Geometry check sheet. Reference: drawing and pictorial views, mm from the part's lowest x, y, z. Give positions to 0.01 mm unless a question says otherwise; leave off trailing zeros. Loops run counter-clockwise (first coordinate to the right, second up) from the corner with the lowest first, then second, coordinate; pieces in that order, holes last. Notation, with made-up numbers: M 59.5,87.25 L 101.5,87.25 A18 ccw 101.5,100.25 Z; hole C -24,13 d9. An arc over 180 degrees is marked long. Put each result on its own line as item: value. Start each with the question number.
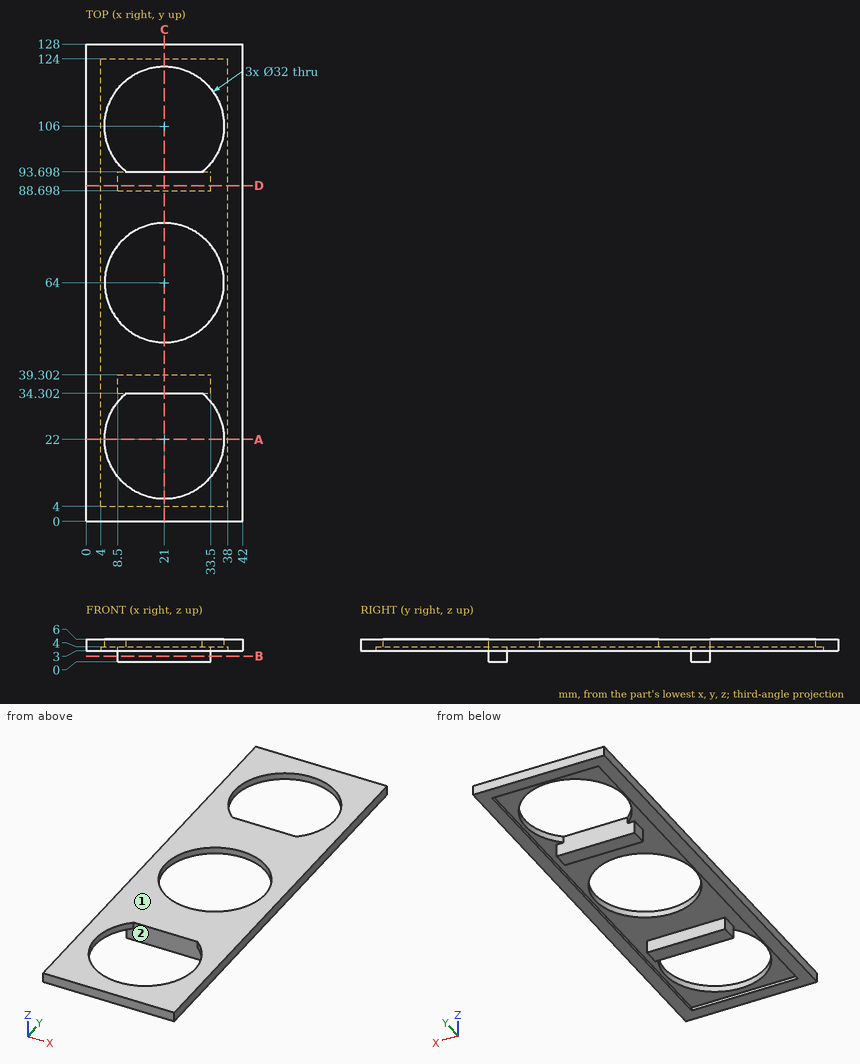
Q1. Section check D-D, the plane y = 90. Record the cut outline in (x, z), then the cut area to 3 significant figures.
Q2. Section check C-C, the plane x = 21. Record the cut outline in (y, z), then the cut area to 3 significant figures.
Q3. Depth check by flat-ended pin: P1, Ø10, axis at x = 22, y = 52.5, coming from the -Z side. Enter the tip coordinate at first touch or a pass-through.
Q4. Section check B-B, the plane z = 1.5. Record the cut outline in (x, y).
Q5. Thickness scan on line 1 along Y through (x, z) = (21, 4.5); line 2 along Y through (x, z) = (29, 3.05); line 3 along Y through (x, z) = (9, 2.05). Record the ranges inside material, lowest first. Write a range as [from, to].
Q6. Section check A-A, the plane y = 22. Record the cut outline in (x, z), then the cut area to 3 significant figures.
Q7. Mould release check, pull along Y, two halves, no side actions. Record for the marked faces 1 and 2: pulls with the +Y half, pulls with the -Y half, needs draft (parallel to the pull), parting line crosses it, or undercut.
Found:
1. outline: M 0,3 L 4,3 L 4,4 L 8.5,4 L 8.5,0 L 33.5,0 L 33.5,4 L 38,4 L 38,3 L 42,3 L 42,6 L 0,6 Z
1. area: 192 mm^2
2. outline: M 0,3 L 4,3 L 4,4 L 6,4 L 6,6 L 0,6 Z; M 34.3,0 L 39.3,0 L 39.3,4 L 48,4 L 48,6 L 34.3,6 Z; M 80,4 L 88.7,4 L 88.7,0 L 93.7,0 L 93.7,6 L 80,6 Z; M 122,4 L 124,4 L 124,3 L 128,3 L 128,6 L 122,6 Z
2. area: 127 mm^2
3. P1: stops at z = 4
4. outline: M 8.5,34.3 L 33.5,34.3 L 33.5,39.3 L 8.5,39.3 Z; M 8.5,88.7 L 33.5,88.7 L 33.5,93.7 L 8.5,93.7 Z
5. line 1: y = [0, 6], [34.3, 48], [80, 93.7], [122, 128]
5. line 2: y = [0, 4], [34.3, 39.3], [88.7, 93.7], [124, 128]
5. line 3: y = [34.3, 39.3], [88.7, 93.7]
6. outline: M 0,3 L 4,3 L 4,4 L 5,4 L 5,6 L 0,6 Z; M 37,4 L 38,4 L 38,3 L 42,3 L 42,6 L 37,6 Z
6. area: 28.0 mm^2
7. face 1: needs draft
7. face 2: undercut
